Autodesk Inventor part; units mm, degrees
ref_plane "YZ Plane" through (0, 0, 0) normal (1, 0, 0) x (0, 1, 0)
ref_plane "XZ Plane" through (0, 0, 0) normal (0, 1, 0) x (-1, 0, 0)
ref_plane "XY Plane" through (0, 0, 0) normal (0, 0, 1) x (1, 0, 0)
sketch "Sketch1" plane through (0, 0, 0) normal (0, 0, 1) x (1, 0, 0)
  line L0 (-8, 8) -> (8, 8)
  line L1 (8, 8) -> (8, -8)
  line L2 (8, -8) -> (-8, -8)
  line L3 (-8, -8) -> (-8, 8)
  point P0 (0, 0)
  dimension "d0" = 16
  dimension "d1" = 16
  dimension "d2" = 8
  dimension "d3" = 8
extrude "Extrusion1" add sketch "Sketch1" along normal blind 9.6
shell "Shell1" thickness 1.5 removed faces 1 at (-2.6667, 2.6667, 0)
sketch "Sketch2" plane through (0, 0, 9.6) normal (0, 0, 1) x (1, 0, 0)
  circle A0 centre (4, -4) radius 2.5
  line L0 (8, 8) -> (8, -8)
  line L1 (8, -8) -> (-8, -8)
  dimension "d7" = 5
  dimension "d10" = 4
  dimension "d11" = 4
extrude "Extrusion2" add sketch "Sketch2" along normal blind 1.6
sketch "Sketch3" plane through (6.5, -6.5, 8.1) normal (0, 0, -1) x (-1, 0, 0)
  circle A0 centre (2.5, 2.5) radius 2.5
  circle A1 centre (2.5, 2.5) radius 1.2
  point P0 (6.5, 6.5)
  dimension "d18" = 2.4
extrude "Extrusion3" cut sketch "Sketch3" against normal blind 1.6 contours A1
pattern_linear "Rectangular Pattern1" count 2 spacing 8 along (0, 1, 0) count 2 spacing 8 along (-1, 0, 0) of "Extrusion2", "Extrusion3"
sketch "Sketch4" plane through (6.5, -6.5, 8.1) normal (0, 0, -1) x (-1, 0, 0)
  circle A0 centre (2.5, 10.5) radius 1.2
  circle A1 centre (2.5, 2.5) radius 1.2
  line L0 (0, 13) -> (0, 0)
  line L1 (0, 0) -> (13, 0)
  circle A2 centre (6.5, 6.5) radius 3.15
  circle A3 centre (6.5, 6.5) radius 2.5
  point P0 (6.5, 6.5)
  dimension "d21" = 6.5
  dimension "d22" = 6.5
  dimension "d23" = 10.5
  dimension "d24" = 2.5
  dimension "d25" = 5
  dimension "d26" = 6.3
extrude "Extrusion4" add sketch "Sketch4" along normal up to surface (8.1 mm away) contours A2
pattern_of_one "Rectangular Pattern2"
equation "\"d0\" = 0.8 * WIDTH"
equation "\"d1\" = 0.8 * LENGTH"
equation "\"d4\" = HEIGHT"
equation "\"d21\" = 0.5 * d23 + 0.5 * d24"
equation "\"d22\" = d21"
equation "\"WIDTH\" = 2"
equation "\"HEIGHT\" = 9.6"
properties part number "3003" material "Steel"
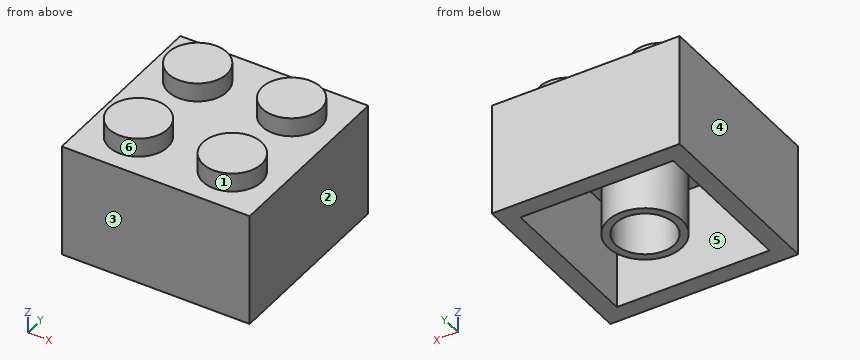
Geometry check sheet. Reference: the model listing, model coordinates, mm. Face numbers are marked on the shaded views. A direction names the side the tool comes from. Round coordinates to 2 decimals unless told otherwise and drop trailing zeros. Loops run counter-clockwise (first coordinate to the right, second up) from the corner with the lowest first, then second, coordinate; pieces in that order, holes last.
Item 1: Cross-section at D-D on y = -4. Record the boundary of the cut face in (x, z).
Item 2: Mould release check, pull along Y, two halves, no side actions. Record for the marked faces 1, 2 and 3: pulls with the +Y half, pulls with the -Y half, needs draft (parallel to the pull), parting line crosses it, or undercut.
Item 3: Access from +Z, -Z, +X, -X, +Y, -Y to the whole of each face (thin tool, end or side, straight path). Record for the marked faces 4, 5 and 6.
Item 4: Cross-section at A-A on z = 6.75. Record the boundary of the cut face in (x, y).
Item 5: Cross-section at B-B on y = 5.5. Record the boundary of the cut face in (x, z), then the cut area to 3 significant figures.
Item 6: Gauge pin test, flat ends, axial feed: pin 1 (3 mm diameter, centred on x = -4, y = 4, fed in from -Z); pin 2 (1 mm diameter, centred on x = 1, y = 3, fed in from +Z). Record the tip position at first contact, or that the pin passes through.
Item 7: Thickness scan on line 1 (Y direction, x = 4, z = 8.6); line 2 (Y direction, x = 0, z = 3); line 3 (X direction, y = -4, z = 7.75). Record the ranges inside material, lowest first.
Answer sheet:
1. outline: (-8, 0) - (-6.5, 0) - (-6.5, 8.1) - (-5.2, 8.1) - (-5.2, 9.7) - (-2.8, 9.7) - (-2.8, 8.1) - (2.8, 8.1) - (2.8, 9.7) - (5.2, 9.7) - (5.2, 8.1) - (6.5, 8.1) - (6.5, 0) - (8, 0) - (8, 9.6) - (6.5, 9.6) - (6.5, 11.2) - (1.5, 11.2) - (1.5, 9.6) - (-1.5, 9.6) - (-1.5, 11.2) - (-6.5, 11.2) - (-6.5, 9.6) - (-8, 9.6) - close
2. face 1: undercut
2. face 2: needs draft
2. face 3: pulls with the -Y half
3. face 4: +Z, -Z, -X, +Y, -Y
3. face 5: -Z
3. face 6: +Z
4. outline: (-8, -8) - (8, -8) - (8, 8) - (-8, 8) - close; circle Ø6.3 at (0, 0); hole (-6.5, -6.5) - (6.5, -6.5) - (6.5, 6.5) - (-6.5, 6.5) - close; hole circle Ø5 at (0, 0)
5. outline: (-8, 0) - (-6.5, 0) - (-6.5, 8.1) - (6.5, 8.1) - (6.5, 0) - (8, 0) - (8, 9.6) - (6, 9.6) - (6, 11.2) - (2, 11.2) - (2, 9.6) - (-2, 9.6) - (-2, 11.2) - (-6, 11.2) - (-6, 9.6) - (-8, 9.6) - close
5. area: 61.1 mm2
6. pin 1: stops at z = 8.1
6. pin 2: stops at z = 9.6
7. line 1: y = -8 to -5.2, -2.8 to 2.8, 5.2 to 8
7. line 2: y = -8 to -6.5, -3.15 to -2.5, 2.5 to 3.15, 6.5 to 8
7. line 3: x = -8 to -6.5, 6.5 to 8
